```python
from build123d import *

# Parameters (mm, degrees)
SKETCH2_W           = 587
SKETCH2_H           = 38
EXTRUDE_THIN1_DEPTH = 38
SKETCH3_W           = 31.95
SKETCH3_H           = 35
BOSS_EXTRUDE1_DEPTH = 100


with BuildPart() as part:
    # Sketch2 → Extrude-Thin1 (new body)
    with BuildSketch(Plane.XY):
        with Locations((-293.5, 19)):
            Rectangle(SKETCH2_W, SKETCH2_H)
    extrude(amount=EXTRUDE_THIN1_DEPTH)

    # Sketch3 → Boss-Extrude1 (add)
    with BuildSketch(Plane.XZ):
        with Locations((-569.525, 19)):
            Rectangle(SKETCH3_W, SKETCH3_H)
    extrude(amount=BOSS_EXTRUDE1_DEPTH)

    # Mirror1: part across plane


with BuildPart() as part_1:
    add(part.part)
    add(part.part.mirror(Plane(origin=(0, 38, 38), x_dir=(0, 0, 1), z_dir=(1, 0, 0))))


solid = part_1.part
```
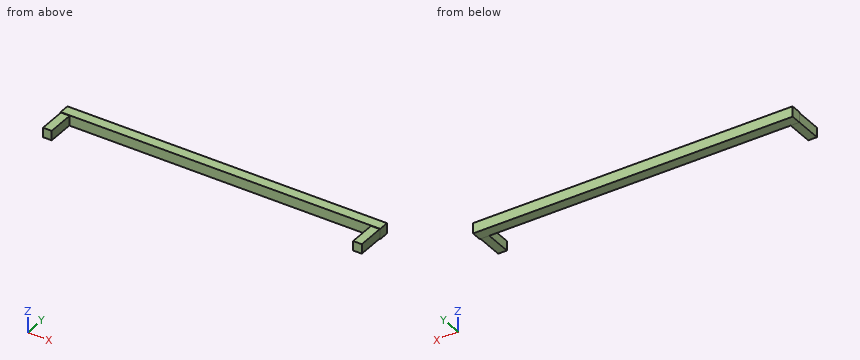
Part model, mm, in its own coordinate system. Round coordinates to 2 decimals unless told otherwise and drop trailing zeros. Write each loop counter-clockwise with the first axis right and the second up, starting at its lowest first coordinate (ties: lowest second). Pieces come first, ordered by that corner, then holes. Notation, with made-up numbers: M 44.5,0 L 102.5,0 A17 ccw 102.5,14 Z; hole C 86,78.5 d2. An arc over 180 degrees is marked long. Answer as CSV lines item,"result". Start each with the question number.
1) Band-saw the part on B-B (z = 24). List the corners of the cut face in (x, y), then the cut area to 3 significant figures.
2) Drop flat-ended pins along their axis: pin 1 (17.5 mm diameter, centred on y = -54.5, z = 20.5, fed in from -X); pin 2 (16 mm diameter, centred on x = -577, y = -38.5, fed in from +Z); pin 3 (3 mm diameter, centred on x = -399, z = 10, fed in from -Y). Give the stop position or say it passes through.
3) Band-saw the part on A-A (y = -46). List the corners of the cut face in (x, z).
4) Drill centre lines: L1, parallel to X at y = -53, z = 4; L2, parallel to Y at x = -240, z = 18.5. Where is each one in solid material? Low to high.
5) Band-saw the part on C-C (x = -360). List the corners of the cut face in (y, z), then the cut area to 3 significant figures.
Worked out:
1,outline,"M -587,0 L -585.5,0 L -585.5,-100 L -553.55,-100 L -553.55,0 L 553.55,0 L 553.55,-100 L 585.5,-100 L 585.5,0 L 587,0 L 587,38 L -587,38 Z"
1,area,"51,000 mm²"
2,pin 1,"x = -585.5"
2,pin 2,"z = 36.5"
2,pin 3,"y = 0"
3,outline,"M -585.5,1.5 L -553.55,1.5 L -553.55,36.5 L -585.5,36.5 Z; M 553.55,1.5 L 585.5,1.5 L 585.5,36.5 L 553.55,36.5 Z"
4,L1,"-585.5 to -553.55, 553.55 to 585.5"
4,L2,"0 to 38"
5,outline,"M 0,0 L 38,0 L 38,38 L 0,38 Z"
5,area,"1,440 mm²"
